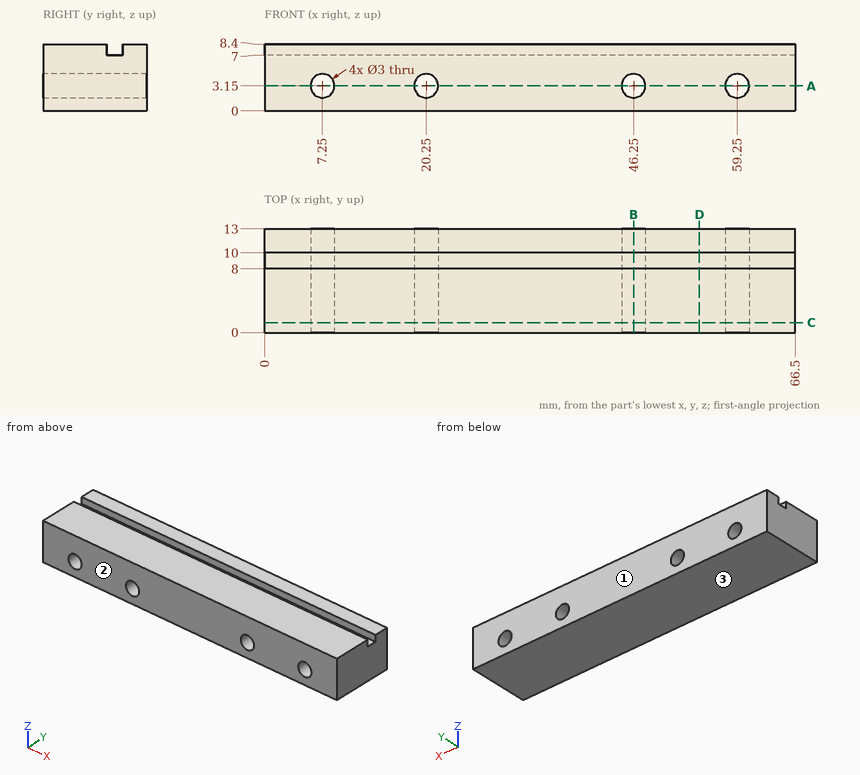
Job drawing, mm, ordinate dimensions from the low corner. One solid piece. Coordinates: 2 decimals unless noted, no trailing zeros. Order: outer loops, then holes, each group sorted by start corner. A loop starts at its lowest first (then second) coordinate and runs counter-clockwise, first axis right, second up. Notation, with made-up numbers: (83, 16.25) -> (96, 16.25) arc R11 ccw to (96, 37.25) -> close; hole circle Ø2 at (6, 83.5). An arc over 180 degrees is marked (long way). Answer in a Markdown table with one row per item. Add a question column.
Q1. Band-saw the part on B-B, the plane x = 46.25. List the corners of the cut face in (y, z), then the cut area to 3 significant figures.
Q2. Band-saw the part on A-A, the plane z = 3.15. List the corners of the cut face in (x, y).
Q3. Band-saw the part on D-D, the plane x = 54.5. List the corners of the cut face in (y, z).
Q4. Band-saw the part on C-C, the plane y = 1.25. List the corners of the cut face in (x, z), then the cut area to 3 significant figures.
Q5. Wall check: line 1 along X through (y, z) = (3.25, 3.15); line 2 along Y through (x, z) = (42, 8.25); line 3 along X through (y, z) = (8.75, 2.25). Give the ranges that are in metal, low to high. Write a range as [from, to].
Q6. Mould opens along Y. For the marked faces 1, 2 and 3 say: +Y half, -Y half, draft (parallel to the pull), parting line (faces both ways), or undercut.
Q7. Drop a flat-ended pin along its axis: pin 1 (1 mm diameter, centred on x = 48, y = 9, fed in from +Z). Give the stop position or say it passes through.
Answers follow:
| question | item | result |
|---|---|---|
| 1 | outline | (0, 0) -> (13, 0) -> (13, 1.65) -> (0, 1.65) -> close; (0, 4.65) -> (13, 4.65) -> (13, 8.4) -> (10, 8.4) -> (10, 7) -> (8, 7) -> (8, 8.4) -> (0, 8.4) -> close |
| 1 | area | 67.4 mm^2 |
| 2 | outline | (0, 0) -> (5.75, 0) -> (5.75, 13) -> (0, 13) -> close; (8.75, 0) -> (18.75, 0) -> (18.75, 13) -> (8.75, 13) -> close; (21.75, 0) -> (44.75, 0) -> (44.75, 13) -> (21.75, 13) -> close; (47.75, 0) -> (57.75, 0) -> (57.75, 13) -> (47.75, 13) -> close; (60.75, 0) -> (66.5, 0) -> (66.5, 13) -> (60.75, 13) -> close |
| 3 | outline | (0, 0) -> (13, 0) -> (13, 8.4) -> (10, 8.4) -> (10, 7) -> (8, 7) -> (8, 8.4) -> (0, 8.4) -> close |
| 4 | outline | (0, 0) -> (66.5, 0) -> (66.5, 8.4) -> (0, 8.4) -> close; hole circle Ø3 at (7.25, 3.15); hole circle Ø3 at (20.25, 3.15); hole circle Ø3 at (46.25, 3.15); hole circle Ø3 at (59.25, 3.15) |
| 4 | area | 530 mm^2 |
| 5 | line 1 | [0, 5.75], [8.75, 18.75], [21.75, 44.75], [47.75, 57.75], [60.75, 66.5] |
| 5 | line 2 | [0, 8], [10, 13] |
| 5 | line 3 | [0, 6.05], [8.45, 19.05], [21.45, 45.05], [47.45, 58.05], [60.45, 66.5] |
| 6 | face 1 | +Y half |
| 6 | face 2 | -Y half |
| 6 | face 3 | draft |
| 7 | pin 1 | z = 7 |
